from build123d import *

# Parameters (mm, degrees)
F1_DEPTH  = 1000
F2_DEPTH  = 900
F3_DEPTH  = 800
F4_DEPTH  = 700
F5_DEPTH  = 600
F6_DEPTH  = 500
F7_DEPTH  = 400
F8_DEPTH  = 300
F9_DEPTH  = 200
F0_W      = 100
F0_H      = 100
F10_DEPTH = 100


with BuildPart() as f1:
    # F0 (on Top) → F1 (new body)
    with BuildSketch(Plane.XY):
        Polygon((900, 900), (900, 0), (1000, 0), (1000, 1000), (0, 1000), (0, 900), align=None)
    extrude(amount=F1_DEPTH)

    # F0 (on Top) → F2 (join)
    with BuildSketch(Plane.XY):
        Polygon((800, 800), (800, 0), (900, 0), (900, 900), (0, 900), (0, 800), align=None)
    extrude(amount=F2_DEPTH)

    # F0 (on Top) → F3 (join)
    with BuildSketch(Plane.XY):
        Polygon((700, 700), (700, 0), (800, 0), (800, 800), (0, 800), (0, 700), align=None)
    extrude(amount=F3_DEPTH)

    # F0 (on Top) → F4 (join)
    with BuildSketch(Plane.XY):
        Polygon((600, 600), (600, 0), (700, 0), (700, 700), (0, 700), (0, 600), align=None)
    extrude(amount=F4_DEPTH)

    # F0 (on Top) → F5 (join)
    with BuildSketch(Plane.XY):
        Polygon((500, 500), (500, 0), (600, 0), (600, 600), (0, 600), (0, 500), align=None)
    extrude(amount=F5_DEPTH)

    # F0 (on Top) → F6 (join)
    with BuildSketch(Plane.XY):
        Polygon((400, 400), (400, 0), (500, 0), (500, 500), (0, 500), (0, 400), align=None)
    extrude(amount=F6_DEPTH)

    # F0 (on Top) → F7 (join)
    with BuildSketch(Plane.XY):
        Polygon((300, 300), (300, 0), (400, 0), (400, 400), (0, 400), (0, 300), align=None)
    extrude(amount=F7_DEPTH)

    # F0 (on Top) → F8 (join)
    with BuildSketch(Plane.XY):
        Polygon((200, 200), (200, 0), (300, 0), (300, 300), (0, 300), (0, 200), align=None)
    extrude(amount=F8_DEPTH)

    # F0 (on Top) → F9 (join)
    with BuildSketch(Plane.XY):
        Polygon((100, 100), (100, 0), (200, 0), (200, 200), (0, 200), (0, 100), align=None)
    extrude(amount=F9_DEPTH)

    # F0 (on Top) → F10 (join)
    with BuildSketch(Plane.XY):
        with Locations((50, 50)):
            Rectangle(F0_W, F0_H)
    extrude(amount=F10_DEPTH)


solid = f1.part
Design review of the part built by this model. Coordinates are the model's own, in mm. A direction names the side the tool comes from. Round coordinates to 2 decimals unless told otherwise and drop trailing zeros. Order: outer loops, then holes, each group sorted by start corner. A loop starts at its lowest first (then second) coordinate and runs counter-clockwise, first axis right, second up.
1) Consider section A-A (x = 776). State the section outline as (y, z) points.
The answers:
outline: (0, 0) - (1000, 0) - (1000, 1000) - (900, 1000) - (900, 900) - (800, 900) - (800, 800) - (0, 800) - close
2) Clearance check with a flat-ended pin moving along its axis: pin 1 Ø6 at (x, y) = (291.5, 239) entering from +Z. State where the tip first meets the part, or that it passes through.
The answers:
pin 1: stops at z = 300
3) Consider section B-B (y = 451). State the section outline as (x, z) points.
The answers:
outline: (0, 0) - (1000, 0) - (1000, 1000) - (900, 1000) - (900, 900) - (800, 900) - (800, 800) - (700, 800) - (700, 700) - (600, 700) - (600, 600) - (500, 600) - (500, 500) - (0, 500) - close
4) For L1, parallel to Z at x = 306, y = 307; L2, parallel to Y at x = 259.5, z = 454.5; L3, parallel to Z at x = 681, y = 111, list the stretches that pass through material, from the lowest coordinate up.
The answers:
L1: z = 0 to 400
L2: y = 400 to 1000
L3: z = 0 to 700
5) Consider section C-C (z = 470). State the section outline as (x, y) points, plus the area to 3 significant figures.
The answers:
outline: (0, 400) - (400, 400) - (400, 0) - (1000, 0) - (1000, 1000) - (0, 1000) - close
area: 840,000 mm2
6) Machinability: for faces 1 (the flat face through (0, 604, 382)), 2 (the flat face through (181, 219, 300)), which of the approach directions +Z, -Z, +X, -X, +Y, -Y give a long, thin tool a straight path to every point of the face, cutting with its end or side? Answer none if there is none.
The answers:
face 1: +Z, -Z, -X, +Y, -Y
face 2: +Z, -X, -Y
